Drawing for the job (mm, zero at the part's lowest x, y, z). Coordinates: 2 decimals unless noted, no trailing zeros. Loops run counter-clockwise (first coordinate to the right, second up) from the corner with the lowest first, then second, coordinate; pieces in that order, holes last. Notation, with made-up numbers: (51, -8) -> (91, -8) arc R25 cw to (91, 14) -> close; hole circle Ø7 at (-36.75, 72). An arc over 180 degrees is marked (long way). Write item = value, one per line. Start each with the question number.
(1) Band-saw the part on A-A (y = 2.05). Write the cut outline in (x, z), and give its area (3 significant figures).
(2) Flat gauge pins, fed straight in: P1, Ø2, axis at x = 32, y = 3, coming from the -Z side; P2, Ø1.5, axis at y = 2.5, z = 82.5, coming from the +X side; P3, Ø2.5, axis at x = 2.5, y = 3, coming from the +Z side; P4, Ø2.5, axis at x = 3.5, y = 3.5, coming from the -Z side. Where does each tip first touch, or does it go through?
(3) Band-saw the part on B-B (z = 10). Write the cut outline in (x, y).
(4) Drill centre line: line 1 (X direction, y = 4.05, z = 12.5). Where is it in solid material? Low to high. Write a range as from..to.
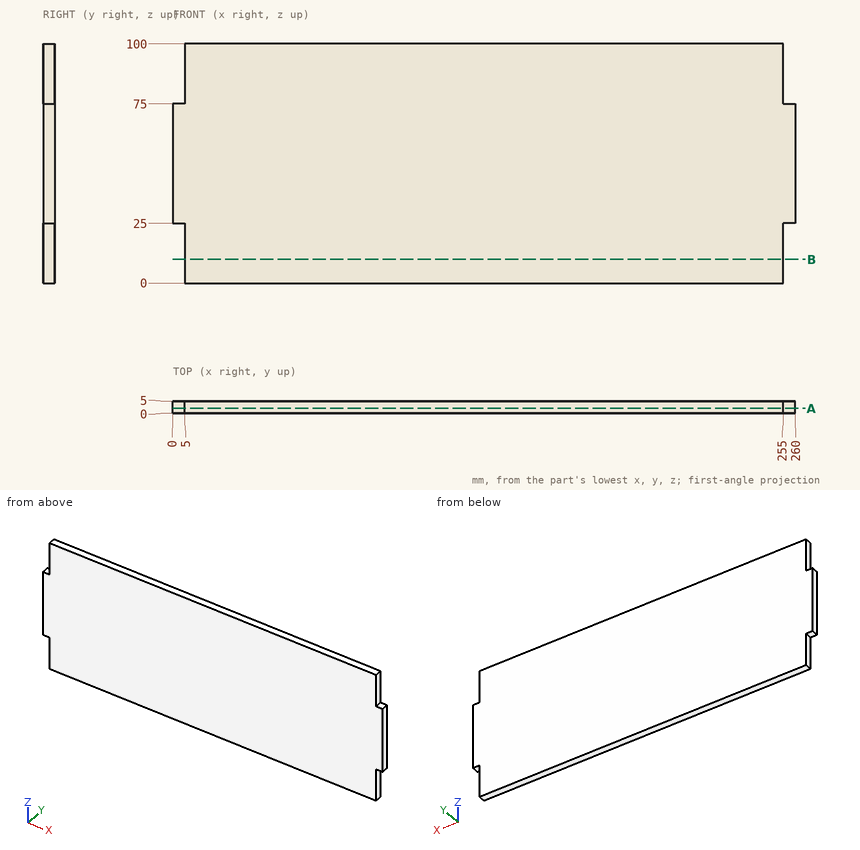
Findings below:
q1.outline = (0, 25) -> (5, 25) -> (5, 0) -> (255, 0) -> (255, 25) -> (260, 25) -> (260, 75) -> (255, 75) -> (255, 100) -> (5, 100) -> (5, 75) -> (0, 75) -> close
q1.area = 25,500 mm²
q2.P1 = 0
q2.P2 = 255
q2.P3 = 75
q2.P4 = 25
q3.outline = (5, 0) -> (255, 0) -> (255, 5) -> (5, 5) -> close
q4.line_1 = 5..255
